Geometry check sheet. Reference: the model listing, model coordinates, mm. A direction names the side the tool comes from. Coordinates: 2 decimals unless noted, no trailing zeros. Order: outer loops, then holes, each group sorted by start corner. A loop starts at its lowest first (then second) coordinate and runs counter-clockwise, first axis right, second up.
```python
from build123d import *

# Parameters (mm, degrees)
SKETCH_1_W          = 170
SKETCH_1_H          = 45
SKETCH_1_R          = 2
SKETCH_1_R_2        = 2.1
EXTRUDE_1_DEPTH     = 4
CUT_EXTRUDE_1_DEPTH = 4
CUT_EXTRUDE_2_DEPTH = 4
FILLET_1_R          = 2


with BuildPart() as part:
    # 草图1 → 凸台-拉伸1 (new body)
    with BuildSketch(Plane(origin=(0, 0, 0), x_dir=(1, 0, 0), z_dir=(0, 1, 0))):
        with Locations((85, 22.5)):
            Rectangle(SKETCH_1_W, SKETCH_1_H)
        with Locations(Location((10, 35, 0), (0, 0, 270))):
            Circle(SKETCH_1_R, mode=Mode.SUBTRACT)
        with Locations(Location((10, 10, 0), (0, 0, 270))):
            Circle(SKETCH_1_R, mode=Mode.SUBTRACT)
        with Locations(Location((160, 10, 0), (0, 0, 270))):
            Circle(SKETCH_1_R, mode=Mode.SUBTRACT)
        with Locations(Location((160, 35, 0), (0, 0, 270))):
            Circle(SKETCH_1_R, mode=Mode.SUBTRACT)
        with Locations(Location((37.5, 35, 0), (0, 0, 270))):
            Circle(SKETCH_1_R_2, mode=Mode.SUBTRACT)
        with Locations(Location((37.5, 10, 0), (0, 0, 270))):
            Circle(SKETCH_1_R_2, mode=Mode.SUBTRACT)
        with Locations(Location((132.5, 10, 0), (0, 0, 270))):
            Circle(SKETCH_1_R_2, mode=Mode.SUBTRACT)
        with Locations(Location((132.5, 35, 0), (0, 0, 270))):
            Circle(SKETCH_1_R_2, mode=Mode.SUBTRACT)
    extrude(amount=EXTRUDE_1_DEPTH)

    # 草图4 → 切除-拉伸1 (cut)
    with BuildSketch(Plane(origin=(0, 4, 0), x_dir=(1, 0, 0), z_dir=(0, 1, 0))):
        Polygon((0, 38.909451479), (6, 45), (0, 45), align=None)
        Polygon((170, 39), (164, 45), (170, 45), align=None)
    extrude(amount=-CUT_EXTRUDE_1_DEPTH, mode=Mode.SUBTRACT)

    # 草图5 → 切除-拉伸2 (cut)
    with BuildSketch(Plane.XZ):
        Polygon((47.5, -5), (47.5, -40), (73.75, -5), align=None)
        Polygon((53.75, -40), (80, -5), (80, -40), align=None)
        Polygon((90, -5), (90, -40), (116.25, -40), align=None)
        Polygon((96.25, -5), (122.5, -5), (122.5, -40), align=None)
    extrude(amount=-CUT_EXTRUDE_2_DEPTH, mode=Mode.SUBTRACT)

    # 圆角1
    fillet_1_edges = [part.edges().sort_by_distance(p)[0] for p in [
        (80, 2, -5),
        (53.75, 2, -40),
        (80, 2, -40),
        (90, 2, -40),
        (116.25, 2, -40),
        (90, 2, -5),
        (122.5, 2, -5),
        (96.25, 2, -5),
        (122.5, 2, -40),
        (47.5, 2, -40),
        (73.75, 2, -5),
        (47.5, 2, -5),
    ]]
    fillet(fillet_1_edges, radius=FILLET_1_R)


solid = part.part
```
Item 1: Thickness scan on line 1 along Z through (x, y) = (160, 2.25); line 2 along Z through (x, y) = (132.5, 1.75); line 3 along X through (y, z) = (1.4, -18.5) (3 decimals). Record the ranges inside material, lowest first.
Item 2: Sectioned sample at B-B (x = 160). Record the cut outline in (y, z), and give its area (3 significant figures).
Item 3: Release check for a two-part mould opening along Z. For faces 1 (the face through (12, 2, -10)), 2 (the face through (84, 2, -45)), 3 (the face through (84, 0, -23)) record: pulls with the +Z half, pulls with the -Z half, needs draft (parallel to the pull), parting line crosses it, or undercut.
Item 4: Tool access check on faces 4 (the face through (114.05, 2.03, -38.87)), 5 (the face through (84, 2, 0)). Record the directions out of +Z, -Z, +X, -X, +Y, -Y that give a thin tool (end or side, any length) a straight path to the whole face; none if there is none.
Item 5: Sectioned sample at C-C (y = 3.4). Give the number of separate pieces and of enclosed holes in the cut face, and give its area (3 significant figures).
Item 6: Sectioned sample at A-A (x = 37.5). Record the cut outline in (y, z), and give its area (3 significant figures).
Geometry check:
1. line 1: z = -45 to -37, -33 to -12, -8 to 0
1. line 2: z = -45 to -37.1, -32.9 to -12.1, -7.9 to 0
1. line 3: x = 0 to 47.5, 63.625 to 69.875, 80 to 90, 100.125 to 106.375, 122.5 to 170
2. outline: (0, -45) - (4, -45) - (4, -37) - (0, -37) - close; (0, -33) - (4, -33) - (4, -12) - (0, -12) - close; (0, -8) - (4, -8) - (4, 0) - (0, 0) - close
2. area: 148 mm2
3. face 1: undercut
3. face 2: pulls with the -Z half
3. face 3: needs draft
4. face 4: +Y, -Y
4. face 5: +Z, +X, -X, +Y, -Y
5. separate pieces: 1
5. enclosed holes: 12
5. area: 5,720 mm2
6. outline: (0, -45) - (4, -45) - (4, -37.1) - (0, -37.1) - close; (0, -32.9) - (4, -32.9) - (4, -12.1) - (0, -12.1) - close; (0, -7.9) - (4, -7.9) - (4, 0) - (0, 0) - close
6. area: 146 mm2
